from build123d import *

# Parameters (mm, degrees)
F0_W     = 500
F0_H     = 350
F0_R     = 3
F0_R_2   = 2.5
F0_W_2   = 330
F0_H_2   = 12
F1_DEPTH = 20
F2_DEPTH = 9
F3_DEPTH = 20


# Not quite as in the source:
# - a feature names something its author has since deleted; it is built from what else it names


with BuildPart() as f1:
    # F0 (on Top) → F1 (new body)
    with BuildSketch(Plane.XY):
        with Locations((250, 175)):
            Rectangle(F0_W, F0_H)
        with Locations((107, 65)):
            Circle(F0_R, mode=Mode.SUBTRACT)
        with Locations((123, 65)):
            Circle(F0_R, mode=Mode.SUBTRACT)
        with Locations((107, 135)):
            Circle(F0_R, mode=Mode.SUBTRACT)
        with Locations((123, 135)):
            Circle(F0_R, mode=Mode.SUBTRACT)
        with Locations((170, 42.5)):
            Circle(F0_R, mode=Mode.SUBTRACT)
        with Locations((245, 42.5)):
            Circle(F0_R, mode=Mode.SUBTRACT)
        with Locations((123.3851659298, 256.5)):
            Circle(F0_R_2, mode=Mode.SUBTRACT)
        with Locations((123.4573769569, 298.5)):
            Circle(F0_R_2, mode=Mode.SUBTRACT)
        with Locations((170, 157.5)):
            Circle(F0_R, mode=Mode.SUBTRACT)
        with Locations((245, 157.5)):
            Circle(F0_R, mode=Mode.SUBTRACT)
        with Locations((320, 42.5)):
            Circle(F0_R, mode=Mode.SUBTRACT)
        with Locations((320, 69)):
            Rectangle(F0_W_2, F0_H_2, mode=Mode.SUBTRACT)
        with Locations((320, 131)):
            Rectangle(F0_W_2, F0_H_2, mode=Mode.SUBTRACT)
        with Locations((395, 42.5)):
            Circle(F0_R, mode=Mode.SUBTRACT)
        with Locations((470, 42.5)):
            Circle(F0_R, mode=Mode.SUBTRACT)
        with Locations((320, 157.5)):
            Circle(F0_R, mode=Mode.SUBTRACT)
        with Locations((395, 157.5)):
            Circle(F0_R, mode=Mode.SUBTRACT)
        with Locations((470, 157.5)):
            Circle(F0_R, mode=Mode.SUBTRACT)
        with Locations((478.6148340702, 256.5)):
            Circle(F0_R_2, mode=Mode.SUBTRACT)
        with Locations((478.5426230431, 298.5)):
            Circle(F0_R_2, mode=Mode.SUBTRACT)
        with Locations((320, 131)):
            Rectangle(F0_W_2, F0_H_2)
        with Locations((245, 157.5)):
            Circle(F0_R)
        with Locations((395, 157.5)):
            Circle(F0_R)
        with Locations((470, 42.5)):
            Circle(F0_R)
        with Locations((395, 42.5)):
            Circle(F0_R)
        with Locations((320, 42.5)):
            Circle(F0_R)
        with Locations((170, 42.5)):
            Circle(F0_R)
        with Locations((245, 42.5)):
            Circle(F0_R)
        with Locations((123, 65)):
            Circle(F0_R)
        with Locations((107, 65)):
            Circle(F0_R)
        with Locations((123, 135)):
            Circle(F0_R)
        with Locations((170, 157.5)):
            Circle(F0_R)
        with Locations((320, 157.5)):
            Circle(F0_R)
        with Locations((470, 157.5)):
            Circle(F0_R)
        with Locations((107, 135)):
            Circle(F0_R)
        with Locations((478.5426230431, 298.5)):
            Circle(F0_R_2)
        with Locations((478.6148340702, 256.5)):
            Circle(F0_R_2)
        with Locations((123.4573769569, 298.5)):
            Circle(F0_R_2)
        with Locations((123.3851659298, 256.5)):
            Circle(F0_R_2)
        with Locations((320, 69)):
            Rectangle(F0_W_2, F0_H_2)
    extrude(amount=-F1_DEPTH)

    # F0 (on Top) → F2 (cut)
    with BuildSketch(Plane.XY):
        with Locations((320, 131)):
            Rectangle(F0_W_2, F0_H_2)
        with Locations((320, 69)):
            Rectangle(F0_W_2, F0_H_2)
    extrude(amount=-F2_DEPTH, mode=Mode.SUBTRACT)

    # F0 (on Top) → F3 (cut)
    with BuildSketch(Plane.XY):
        with Locations((170, 42.5)):
            Circle(F0_R)
        with Locations((245, 42.5)):
            Circle(F0_R)
        with Locations((320, 42.5)):
            Circle(F0_R)
        with Locations((395, 42.5)):
            Circle(F0_R)
        with Locations((470, 42.5)):
            Circle(F0_R)
        with Locations((470, 157.5)):
            Circle(F0_R)
        with Locations((395, 157.5)):
            Circle(F0_R)
        with Locations((320, 157.5)):
            Circle(F0_R)
        with Locations((245, 157.5)):
            Circle(F0_R)
        with Locations((170, 157.5)):
            Circle(F0_R)
        with Locations((107, 135)):
            Circle(F0_R)
        with Locations((123, 135)):
            Circle(F0_R)
        with Locations((123, 65)):
            Circle(F0_R)
        with Locations((107, 65)):
            Circle(F0_R)
        with Locations((478.5426230431, 298.5)):
            Circle(F0_R_2)
        with Locations((478.6148340702, 256.5)):
            Circle(F0_R_2)
        with Locations((123.3851659298, 256.5)):
            Circle(F0_R_2)
        with Locations((123.4573769569, 298.5)):
            Circle(F0_R_2)
    extrude(amount=-F3_DEPTH, mode=Mode.SUBTRACT)


solid = f1.part
Design review of the part built by this model. Coordinates are the model's own, in mm. A direction names the side the tool comes from. Give positions to 0.01 mm unless a question says otherwise; leave off trailing zeros. Loops run counter-clockwise (first coordinate to the right, second up) from the corner with the lowest first, then second, coordinate; pieces in that order, holes last. Notation, with made-up numbers: (39.25, -5) -> (68.25, -5) arc R19 ccw to (68.25, 31) -> close; hole circle Ø11 at (-19, -28). An arc over 180 degrees is marked (long way). One line per question, with ' | ' between items. Start each with the question number.
(1) We need section B-B (x = 225). State the section outline as (y, z) points, and give its area (3 significant figures).
(2) Draft analysis for pull direction Y (two halves, no side actions). For faces 3 (the face through (247, 0, -10)), 4 (the face through (318, 131, -9)), 5 (the face through (247, 177, 0)), state which applies: +Y half, -Y half, draft (parallel to the pull), parting line (faces both ways), or undercut.
(3) For line 1 (Y direction, x = 245, z = -4.5); line 2 (Y direction, x = 301, z = -5.5); line 3 (X direction, y = 157.5, z = -7.25), list the stretches that pass through material, from the lowest coordinate up.
(4) We need section A-A (z = -5.25). State how many separate pieces and enclosed holes the cut face has, and give its area (3 significant figures).
(5) Insertion check: P1, Ø3.5, axis at x = 170, y = 157.5, coming from the +Z side. The pin has a flat end and moves straight along its axis. Give the tip position at first contact, or say it passes through.
(6) For faces 1 (the face through (318, 69, -9)), 2 (the face through (247, 177, -20)), list the 3-axis set-ups (+Z, -Z, +X, -X, +Y, -Y) from which the entire face can be reached by the end or side of a thin tool; tool diameter is ignored.
The answers:
1) outline: (0, -20) -> (350, -20) -> (350, 0) -> (137, 0) -> (137, -9) -> (125, -9) -> (125, 0) -> (75, 0) -> (75, -9) -> (63, -9) -> (63, 0) -> (0, 0) -> close | area: 6,780 mm^2
2) face 3: -Y half | face 4: undercut | face 5: draft
3) line 1: y = 0 to 39.5, 45.5 to 63, 75 to 125, 137 to 154.5, 160.5 to 350 | line 2: y = 0 to 63, 75 to 125, 137 to 350 | line 3: x = 0 to 167, 173 to 242, 248 to 317, 323 to 392, 398 to 467, 473 to 500
4) separate pieces: 1 | enclosed holes: 20 | area: 167,000 mm^2
5) P1: passes through
6) face 1: +Z | face 2: -Z, +X, -X, +Y, -Y
